Input: part model. Units: mm. Frame: model coordinates. Face numbers are marked on the shaded views. A direction names the side the tool comes from. Give positions to 0.01 mm unless a question says otherwise; leave off trailing zeros. Write each loop counter-clockwise with the first axis right and the second up, starting at its lowest first coordinate (ties: lowest second). Pieces come first, ordered by that corner, then holes. Notation, with made-up numbers: (-25, 28) -> (9, 28) arc R15 cw to (9, 34) -> close; hole circle Ø6 at (80.25, 82). An arc over 180 degrees is marked (long way). Answer as a JSON object with one key per item and string values. Group by question number.
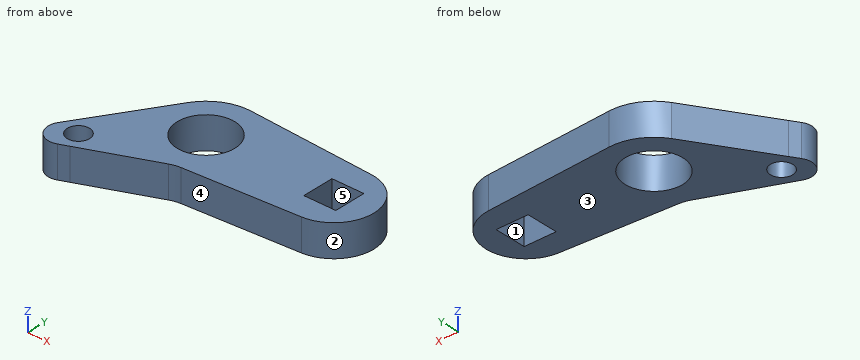
from build123d import *

# Parameters (mm, degrees)
SKETCH_1_R      = 6
SKETCH_1_R_2    = 3.5
SKETCH_1_R_3    = 15
SKETCH_1_R_4    = 9
SKETCH_1_R_5    = 12.5
SKETCH_1_W      = 10
SKETCH_1_H      = 10
EXTRUDE_1_DEPTH = 10
FILLET_1_R      = 5
FILLET_2_R      = 10


with BuildPart() as part:
    # Эскиз1 → Бобышка-Вытянуть1 (new body)
    # profile 1 of 7: a face of its own
    with BuildSketch(Plane.XY):
        with BuildLine():
            Line((-12.64490448, 8.068853121), (-28.039295072, -16.056087022))
            ThreePointArc((-28.039295072, -16.056087022), (-21.300228103, -13.523950753), (-16.981333294, -19.283628291))
            ThreePointArc((-16.981333294, -19.283628291), (-17.991282662, -22.615203698), (-20.681131524, -24.825204945))
            Line((-20.681131524, -24.825204945), (3.437235755, -14.814134934))
            Line((3.437235755, -14.814134934), (0.9375, -14.970674459))
            ThreePointArc((0.9375, -14.970674459), (-12.921717676, -7.617690746), (-12.64490448, 8.068853121))
        make_face()
    # profile 2 of 7: a face of its own
    with BuildSketch(Plane.XY):
        with Locations((-22.981333294, -19.283628291)):
            Circle(SKETCH_1_R)
        with Locations((-22.981333294, -19.283628291)):
            Circle(SKETCH_1_R_2, mode=Mode.SUBTRACT)
    # profile 3 of 7: a face of its own
    with BuildSketch(Plane.XY):
        with BuildLine():
            Line((-28.039295072, -16.056087022), (-38.302222156, -32.139380484))
            Line((-38.302222156, -32.139380484), (-20.681131524, -24.825204945))
            ThreePointArc((-20.681131524, -24.825204945), (-27.57759997, -23.140353928), (-28.039295072, -16.056087022))
        make_face()
    # profile 4 of 7: a face of its own
    with BuildSketch(Plane.XY):
        Circle(SKETCH_1_R_3)
        Circle(SKETCH_1_R_4, mode=Mode.SUBTRACT)
    # profile 5 of 7: a face of its own
    with BuildSketch(Plane.XY):
        with BuildLine():
            Line((5.750504492, -13.853941608), (3.437235755, -14.814134934))
            Line((3.437235755, -14.814134934), (40.78125, -12.475562049))
            ThreePointArc((40.78125, -12.475562049), (27.5, 0), (40.78125, 12.475562049))
            Line((40.78125, 12.475562049), (0.9375, 14.970674459))
            ThreePointArc((0.9375, 14.970674459), (10.933034803, 10.269797953), (15, 0))
            ThreePointArc((15, 0), (12.4751266, -8.328938486), (5.750504492, -13.853941608))
        make_face()
    # profile 6 of 7: a face of its own
    with BuildSketch(Plane.XY):
        with Locations((40, 0)):
            Circle(SKETCH_1_R_5)
        with Locations((40, 0)):
            Rectangle(SKETCH_1_W, SKETCH_1_H, mode=Mode.SUBTRACT)
    # profile 7 of 7: a face of its own
    with BuildSketch(Plane.XY):
        with BuildLine():
            Line((0.9375, -14.970674459), (3.437235755, -14.814134934))
            Line((3.437235755, -14.814134934), (5.750504492, -13.853941608))
            ThreePointArc((5.750504492, -13.853941608), (3.390298525, -14.611840264), (0.9375, -14.970674459))
        make_face()
    extrude(amount=EXTRUDE_1_DEPTH)

    # Скругление1
    fillet_1_edges = [part.edges().sort_by_distance(p)[0] for p in [
        (-38.302222156, -32.139380484, 5),
    ]]
    fillet(fillet_1_edges, radius=FILLET_1_R)

    # Скругление2
    fillet_2_edges = [part.edges().sort_by_distance(p)[0] for p in [
        (3.437235755, -14.814134934, 5),
    ]]
    fillet(fillet_2_edges, radius=FILLET_2_R)


solid = part.part
1. Section A-A (x = 40). Return the cut outline in (y, z).
2. Reachability of the marked faces 1 and 2 from +Z, -Z, +X, -X, +Y, -Y: full face, straight path, thin tool, end or side. Return the list, or none.
3. Mould query, pull axis X, two halves, no side actions, for the marked faces 3, 4 and 5. Classes: pulls with the +X half, pulls with the -X half, needs draft (parallel to the pull), parting line crosses it, or undercut.
4. Section B-B (y = 1). Return the cut outline in (x, z).
5. Section C-C (z = 8.75). Return the cut outline in (x, y).
6. Section D-D (x = -4.5). Return the cut outline in (y, z), plus the area to 3 significant figures.
7. Line query: line 1 (X direction, y = -1.5, z = 7.25); line 2 (X direction, y = -7.5, z = 2.75); line 3 (X direction, y = 6, z = 4.75). Output: solid intervals per line, ascending.
8. Contact query for flat-ended pins moving along their axis: pin 1 Ø4 at (y, z) = (5, 5) entering from -X; pin 2 Ø5.5 at (x, y) = (-22.98, -19.28) entering from -Z; pin 3 Ø4 at (x, z) = (-4, 4) entering from -Y; pin 4 Ø3 at (x, z) = (41.5, 4) entering from +Y. Output: stop coordinate, or through.
Working result:
{
 "1": {"outline": "(-12.52, 0) -> (-5, 0) -> (-5, 10) -> (-12.52, 10) -> close; (5, 0) -> (12.52, 0) -> (12.52, 10) -> (5, 10) -> close"},
 "2": {"face 1": "+Z, -Z", "face 2": "+Z, -Z, +X"},
 "3": {"face 3": "needs draft", "face 4": "pulls with the +X half", "face 5": "undercut"},
 "4": {"outline": "(-17.16, 0) -> (-8.94, 0) -> (-8.94, 10) -> (-17.16, 10) -> close; (8.94, 0) -> (35, 0) -> (35, 10) -> (8.94, 10) -> close; (45, 0) -> (52.46, 0) -> (52.46, 10) -> (45, 10) -> close"},
 "5": {"outline": "(-29.75, -18.74) arc R5 ccw to (-23.62, -26.04) -> (1.9, -15.45) arc R10 cw to (5.1, -14.71) -> (40.78, -12.48) arc R12.5 ccw to (40.78, 12.48) -> (0.94, 14.97) arc R15 ccw to (-12.64, 8.07) -> close; hole circle Ø7 at (-22.98, -19.28); hole circle Ø18 at (0, 0); hole (35, -5) -> (45, -5) -> (45, 5) -> (35, 5) -> close"},
 "6": {"outline": "(-18.11, 0) -> (-7.79, 0) -> (-7.79, 10) -> (-18.11, 10) -> close; (7.79, 0) -> (14.31, 0) -> (14.31, 10) -> (7.79, 10) -> close", "area": "168 mm^2"},
 "7": {"line 1": "x = -18.75 to -8.87, 8.87 to 35, 45 to 52.41", "line 2": "x = -22.58 to -4.97, 4.97 to 50", "line 3": "x = -13.97 to -6.71, 6.71 to 50.97"},
 "8": {"pin 1": "stops at x = -15.88", "pin 2": "passes through", "pin 3": "stops at y = -18.73", "pin 4": "stops at y = 12.52"}
}
